Check sheet for the drawn part. Datum: minimum x, y, z corner. Units: mm. Round coordinates to 2 decimals unless told otherwise and drop trailing zeros. Write each loop counter-clockwise with the first axis right and the second up, starting at its lowest first coordinate (ties: lowest second). Pieces come first, ordered by that corner, then holes.
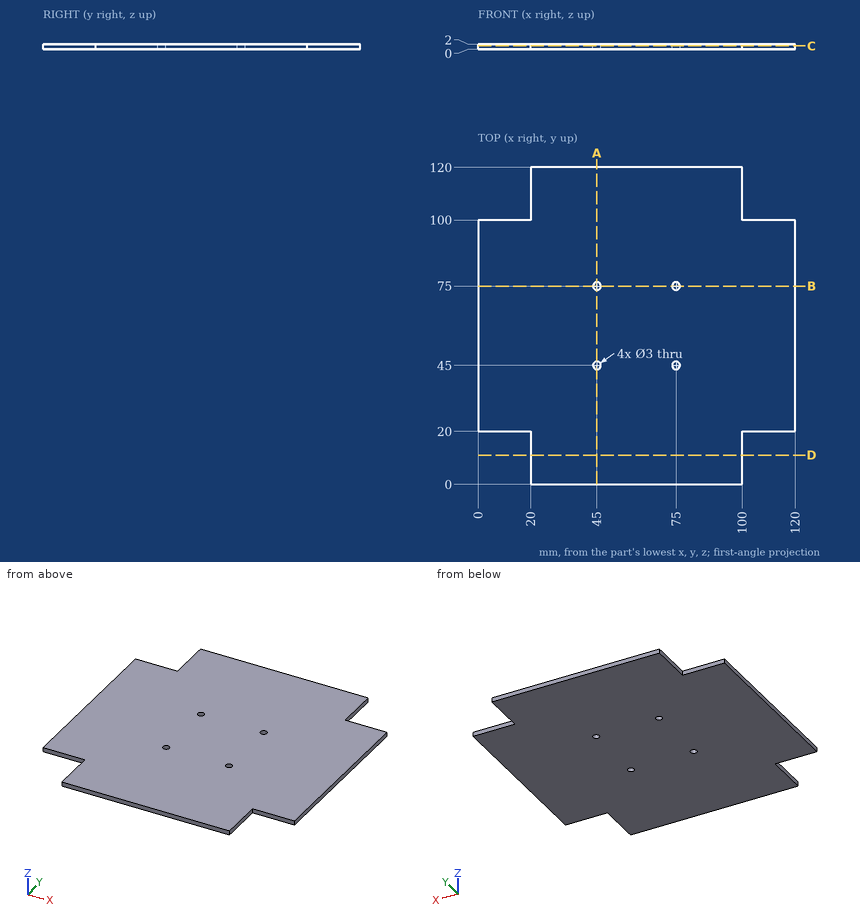
1. Scan lines: line 1 along X through (y, z) = (45, 0.7); line 2 along X through (y, z) = (45.5, 0.35). Record each from-to range of solid material in increasing order.
2. Sectioned sample at D-D, the plane y = 11. Enter the section's corners in (x, z), plus the area to 3 significant figures.
3. Sectioned sample at A-A, the plane x = 45. Enter the section's corners in (y, z).
4. Sectioned sample at C-C, the plane z = 1.25. Enter the section's corners in (x, y).
5. Go/stop test with flat-tipped pins: pin 1 (1 mm diameter, centred on y = 114, z = 1.5, fed in from -X); pin 2 (1 mm diameter, centred on x = 11, z = 0.5, fed in from -Y); pin 3 (1.8 mm diameter, centred on x = 75, y = 75, fed in from +Z); pin 4 (1 mm diameter, centred on y = 111, z = 0.5, fed in from +X). Record where each tip stops, or that it passes through.
Computed values:
1. line 1: x = 0 to 43.5, 46.5 to 73.5, 76.5 to 120
1. line 2: x = 0 to 43.59, 46.41 to 73.59, 76.41 to 120
2. outline: (20, 0) - (100, 0) - (100, 2) - (20, 2) - close
2. area: 160 mm2
3. outline: (0, 0) - (43.5, 0) - (43.5, 2) - (0, 2) - close; (46.5, 0) - (73.5, 0) - (73.5, 2) - (46.5, 2) - close; (76.5, 0) - (120, 0) - (120, 2) - (76.5, 2) - close
4. outline: (0, 20) - (20, 20) - (20, 0) - (100, 0) - (100, 20) - (120, 20) - (120, 100) - (100, 100) - (100, 120) - (20, 120) - (20, 100) - (0, 100) - close; hole circle Ø3 at (45, 45); hole circle Ø3 at (45, 75); hole circle Ø3 at (75, 45); hole circle Ø3 at (75, 75)
5. pin 1: stops at x = 20
5. pin 2: stops at y = 20
5. pin 3: passes through
5. pin 4: stops at x = 100
